from build123d import *

# Parameters (mm, degrees)
F0_R     = 10.5
F1_DEPTH = 14.2875
F2_W     = 170
F2_H     = 29.6946875751
F3_DEPTH = 14.2875
F5_DEPTH = 14.2875


# Not quite as in the source:
# - a length typed as a fraction of an inch, garbled in the dataset ("3 / 203.2 mm" for 3/8 in), is restored
# - a feature names something its author has since deleted; it is built from what else it names


with BuildPart() as f1:
    # F0 (on Top) → F1 (new body)
    with BuildSketch(Plane.XY):
        with BuildLine():
            ThreePointArc((-84.5842045546, -55), (-80.1908062724, -65.6066017178), (-69.5842045546, -70))
            Line((-69.5842045546, -70), (69.5842045546, -70))
            ThreePointArc((69.5842045546, -70), (80.7788298305, -65.363034385), (85.4157954454, -54.1684091091))
            Line((85.4157954454, -54.1684091091), (85.4157954454, 203.1919921827))
            ThreePointArc((85.4157954454, 203.1919921827), (85.0717839963, 205.0145647093), (84.0870871996, 206.5863429094))
            Line((84.0870871996, 206.5863429094), (27.5340619023, 267.7534620916))
            ThreePointArc((27.5340619023, 267.7534620916), (24.0585970267, 269.3552750765), (20.4684194215, 268.030403119))
            Line((20.4684194215, 268.030403119), (13.1258359132, 261.2417016656))
            Line((13.1258359132, 261.2417016656), (26.70323882, 246.556534649))
            Line((26.70323882, 246.556534649), (16.0564927329, 236.7129175415))
            Line((16.0564927329, 236.7129175415), (5.4097466459, 226.8693004341))
            Line((5.4097466459, 226.8693004341), (-8.1676562609, 241.5544674507))
            Line((-8.1676562609, 241.5544674507), (-18.3614984488, 232.1295897903))
            ThreePointArc((-18.3614984488, 232.1295897903), (-19.0801780579, 231.3013565049), (-19.6010257192, 230.336375433))
            Line((-19.6010257192, 230.336375433), (-83.4858385457, 72.7100555545))
            ThreePointArc((-83.4858385457, 72.7100555545), (-84.3070526124, 69.9459705844), (-84.5842045546, 67.0758233641))
            Line((-84.5842045546, 67.0758233641), (-84.5842045546, -55))
        make_face()
        with Locations((-40, 0)):
            Circle(F0_R, mode=Mode.SUBTRACT)
        with Locations((40, 0)):
            Circle(F0_R, mode=Mode.SUBTRACT)
    extrude(amount=F1_DEPTH)

    # F2 (on face) → F3 (join)
    with BuildSketch(Plane(origin=(0, 0, 0), x_dir=(1, 0, 0), z_dir=(0, 0, -1))):
        with BuildLine():
            ThreePointArc((-110.4471534491, -61.8855160475), (-108.982687355, -65.4210499534), (-105.4471534491, -66.8855160475))
            Line((-105.4471534491, -66.8855160475), (-84.5842045546, -66.8855160475))
            Line((-84.5842045546, -66.8855160475), (-84.5842045546, -37.1908284724))
            Line((-84.5842045546, -37.1908284724), (-110.4471534491, -37.1908284724))
            Line((-110.4471534491, -37.1908284724), (-110.4471534491, -61.8855160475))
        make_face()
        with Locations((0.4157954454, -52.0381722599)):
            Rectangle(F2_W, F2_H)
        with BuildLine():
            Line((85.4157954454, -37.1908284724), (85.4157954454, -66.8855160475))
            Line((85.4157954454, -66.8855160475), (106.2211793661, -66.8855160475))
            ThreePointArc((106.2211793661, -66.8855160475), (109.756713272, -65.4210499534), (111.2211793661, -61.8855160475))
            Line((111.2211793661, -61.8855160475), (111.2211793661, -37.1908284724))
            Line((111.2211793661, -37.1908284724), (85.4157954454, -37.1908284724))
        make_face()
        with BuildLine():
            Line((-84.5842045546, 55), (-84.5842045546, 37.1908284724))
            Line((-84.5842045546, 37.1908284724), (85.4157954454, 37.1908284724))
            Line((85.4157954454, 37.1908284724), (85.4157954454, 54.1684091091))
            ThreePointArc((85.4157954454, 54.1684091091), (83.7249684911, 61.287261926), (79.0136510523, 66.8855160475))
            Line((79.0136510523, 66.8855160475), (-78.7348607215, 66.8855160475))
            ThreePointArc((-78.7348607215, 66.8855160475), (-83.0426562208, 61.623449158), (-84.5842045546, 55))
        make_face()
        with BuildLine():
            Line((-110.4471534491, 37.1908284724), (-84.5842045546, 37.1908284724))
            Line((-84.5842045546, 37.1908284724), (-84.5842045546, 55))
            ThreePointArc((-84.5842045546, 55), (-83.0426562208, 61.623449158), (-78.7348607215, 66.8855160475))
            Line((-78.7348607215, 66.8855160475), (-105.4471534491, 66.8855160475))
            ThreePointArc((-105.4471534491, 66.8855160475), (-108.982687355, 65.4210499534), (-110.4471534491, 61.8855160475))
            Line((-110.4471534491, 61.8855160475), (-110.4471534491, 37.1908284724))
        make_face()
        with BuildLine():
            Line((85.4157954454, 54.1684091091), (85.4157954454, 37.1908284724))
            Line((85.4157954454, 37.1908284724), (111.2211793661, 37.1908284724))
            Line((111.2211793661, 37.1908284724), (111.2211793661, 61.8855160475))
            ThreePointArc((111.2211793661, 61.8855160475), (109.756713272, 65.4210499534), (106.2211793661, 66.8855160475))
            Line((106.2211793661, 66.8855160475), (79.0136510523, 66.8855160475))
            ThreePointArc((79.0136510523, 66.8855160475), (83.7249684911, 61.287261926), (85.4157954454, 54.1684091091))
        make_face()
    extrude(amount=F3_DEPTH)

    # F4 (on face) → F5 (join)
    with BuildSketch(Plane.XY.offset(14.2875)):
        with BuildLine():
            Line((-8.2645773549, 49.9606142757), (76.5538805598, 49.9606142757))
            ThreePointArc((76.5538805598, 49.9606142757), (80.0894144658, 51.4250803698), (81.5538805598, 54.9606142757))
            Line((81.5538805598, 54.9606142757), (81.5538805598, 205.2832095857))
            ThreePointArc((81.5538805598, 205.2832095857), (81.2098691107, 207.1057821123), (80.225172314, 208.6775603124))
            Line((80.225172314, 208.6775603124), (26.4943680898, 266.7921967701))
            ThreePointArc((26.4943680898, 266.7921967701), (23.0189032141, 268.3940097551), (19.4287256089, 267.0691377976))
            Line((19.4287256089, 267.0691377976), (13.1258359132, 261.2417016656))
            Line((13.1258359132, 261.2417016656), (26.70323882, 246.556534649))
            Line((26.70323882, 246.556534649), (5.4097466459, 226.8693004341))
            Line((5.4097466459, 226.8693004341), (-8.1676562609, 241.5544674507))
            Line((-8.1676562609, 241.5544674507), (-13.2645773549, 236.8420286205))
            Line((-13.2645773549, 236.8420286205), (-13.2645773549, 54.9606142757))
            ThreePointArc((-13.2645773549, 54.9606142757), (-11.8001112608, 51.4250803698), (-8.2645773549, 49.9606142757))
        make_face()
    extrude(amount=F5_DEPTH)


solid = f1.part
The listing builds one solid part. Answer for the finished solid, in the listing's coordinates (mm). A direction names the side the tool comes from. Round coordinates to 2 decimals unless told otherwise and drop trailing zeros. Write each loop counter-clockwise with the first axis right and the second up, starting at its lowest first coordinate (ties: lowest second). Pieces come first, ordered by that corner, then holes. Notation, with made-up numbers: M 10.25,-9 L 23.25,-9 A7 ccw 23.25,-4 Z; hole C 40,70 d11. An arc over 180 degrees is marked long. Write each question's results on one line, items separated by ' | '. Start each with the question number.
Item 1: For faces 4 (the face through (34, 49.961, 21)), 5 (the face through (-84.584, 7, 7)), 6 (the face through (85.416, 73, 7)), 7 (the face through (-1, -37.191, -7)), 8 (the face through (80.655, -65.485, 7.044)), determine the directions among +Z, -Z, +X, -X, +Y, -Y from which every point of the face is accessible in a straight line to the end or side of a thin tool.
Item 2: A cutting plane is placed at A-A on z = -10. Write down the section's boundary in (x, y).
Item 3: A cutting plane is placed at D-D on x = 33.5. Write down the section's boundary in (y, z) (1 decimal), and give its area (3 significant figures).
Item 4: Flat-ended cylindrical pins translate along their axes: pin 1 Ø20.5 at (x, y) = (-94.5, 58) entering from +Z; pin 2 Ø4.5 at (x, z) = (19.5, -7) entering from +Y; pin 3 Ø9 at (x, y) = (95, -45) entering from +Z; pin 4 Ø1.5 at (x, y) = (-54.5, 151.5) entering from +Z. Find the tip coordinate at first contact, or state that the pin passes through.
Item 5: A cutting plane is placed at B-B on y = 0. Write down the section's boundary in (x, z), and give its area (3 significant figures).
Item 6: Straight lines are drawn through the part: L1, parallel to Y at x = -84, z = -4; L2, parallel to Z at x = 9, y = 109 (3 decimals); L3, parallel to X at y = 59, z = 23.5. For each, find the intervals that lie inside material, in ascending order. Write a range as [from, to].
Item 7: For a pull along X with two mould halves and no side action, classify faces 1 (the face through (-110.447, -50, -7)), 2 (the face through (-1, 52, -14.288)), 3 (the face through (16.206, 236.851, 14.087)) as pulls with the +X half, pulls with the -X half, needs draft (parallel to the pull), parting line crosses it, or undercut.
Item 8: A cutting plane is placed at C-C on z = 6. Write down the section's boundary in (x, y), and give its area (3 significant figures).
Check sheet entries:
1) face 4: +Z, +X, -X, -Y | face 5: +Z, -X, +Y, -Y | face 6: +Z, +X, +Y, -Y | face 7: -Z, +X, -X | face 8: +Z, +X, -Y
2) outline: M -110.45,-61.89 A5 ccw -105.45,-66.89 L 106.22,-66.89 A5 ccw 111.22,-61.89 L 111.22,-37.19 L -110.45,-37.19 Z; M -110.45,37.19 L 111.22,37.19 L 111.22,61.89 A5 ccw 106.22,66.89 L -105.45,66.89 A5 ccw -110.45,61.89 Z
3) outline: M -70,0 L -66.9,0 L -66.9,-14.3 L -37.2,-14.3 L -37.2,0 L -8.2,0 L -8.2,14.3 L -70,14.3 Z; M 8.2,0 L 37.2,0 L 37.2,-14.3 L 66.9,-14.3 L 66.9,0 L 261.3,0 L 261.3,14.3 L 259.2,14.3 L 259.2,28.6 L 50,28.6 L 50,14.3 L 8.2,14.3 Z | area: 8,340 mm²
4) pin 1: z = 14.29 | pin 2: y = 66.89 | pin 3: z = 0 | pin 4: through
5) outline: M -84.58,0 L -50.5,0 L -50.5,14.29 L -84.58,14.29 Z; M -29.5,0 L 29.5,0 L 29.5,14.29 L -29.5,14.29 Z; M 50.5,0 L 85.42,0 L 85.42,14.29 L 50.5,14.29 Z | area: 1,830 mm²
6) L1: [-66.89, -37.19], [37.19, 66.89] | L2: [0, 28.575] | L3: [-13.26, 81.55]
7) face 1: pulls with the -X half | face 2: needs draft | face 3: undercut
8) outline: M -84.58,-55 A15 ccw -69.58,-70 L 69.58,-70 A15.83 ccw 85.42,-54.17 L 85.42,203.19 A5 ccw 84.09,206.59 L 27.53,267.75 A5 ccw 20.47,268.03 L 13.13,261.24 L 26.7,246.56 L 5.41,226.87 L -8.17,241.55 L -18.36,232.13 A5 ccw -19.6,230.34 L -83.49,72.71 A15 ccw -84.58,67.08 Z; hole C -40,0 d21; hole C 40,0 d21 | area: 45,900 mm²
